```python
from build123d import *

# Parameters (mm, degrees)
ESQUISSE1_R = 1.25


with BuildPart() as part:
    # Balayage1: sweep along a path in Esquisse2
    with BuildLine(Plane(origin=(0, 0, 0), x_dir=(1, 0, 0), z_dir=(0, 1, 0))) as balayage1_path:
        Line((0, 0), (0, 5))
        ThreePointArc((0, 5), (-0.732233047, 6.767766953), (-2.5, 7.5))
        Line((-2.5, 7.5), (-25, 7.5))
        ThreePointArc((-25, 7.5), (-26.767766953, 6.767766953), (-27.5, 5))
        Line((-27.5, 5), (-27.5, -10))
        ThreePointArc((-27.5, -10), (-26.767766953, -11.767766953), (-25, -12.5))
        Line((-25, -12.5), (-2.5, -12.5))
        ThreePointArc((-2.5, -12.5), (-0.732233047, -11.767766953), (0, -10))
        Line((0, -10), (0, -5))
    # Esquisse1 → Balayage1 (sweep)
    with BuildSketch(Plane.XY):
        Circle(ESQUISSE1_R)
    sweep(path=balayage1_path.line)


solid = part.part
```
Build history of the part. All positions in model axes, mm. A direction names the side the tool comes from. Round coordinates to 2 decimals unless told otherwise and drop trailing zeros. Write each loop counter-clockwise with the first axis right and the second up, starting at its lowest first coordinate (ties: lowest second). Pieces come first, ordered by that corner, then holes. Notation, with made-up numbers: (43, 23) - (50, 23) arc R12 ccw to (50, 28) - close; hole circle Ø5 at (-22, 75). An arc over 180 degrees is marked (long way). Write each question's results on one line, items separated by ' | '. Start each with the question number.
Item 1: Wall check: L1, parallel to Z at x = -19, y = 0.05; L2, parallel to X at y = -0.1, z = -2.25; L3, parallel to Z at x = -24.5, y = -0.95. Give the ranges that are in metal, low to high. Write a range as [from, to].
Item 2: Saw through at B-B (z = 8). Write the cut outline in (x, y).
Item 3: Saw through at A-A (y = 0). Write the cut outline in (x, z), and give its area (3 significant figures).
Item 4: Saw through at C-C (x = -20). Write the cut outline in (y, z), and give its area (3 significant figures).
Item 5: Drop a flat-ended pin along its axis: P1, Ø1.2, axis at x = -0.5, y = 0.5, coming from the +Z side. Give the stop position or say it passes through.
Item 6: Saw through at D-D (z = 3). Write the cut outline in (x, y), and give its area (3 significant figures).
Item 7: Mould opens along X. For faces 1 (the face through (-13.91, -0.05, -6.25)), 2 (the face through (-13.59, -0.05, 11.25)), 3 (the face through (0, 0, 0)) say: pulls with the +X half, pulls with the -X half, needs draft (parallel to the pull), parting line crosses it, or undercut.
Item 8: Which spindle directions (+Z, -Z, +X, -X, +Y, -Y) get a long thin tool onto all of the face, cutting with end or side? Do faces 4 (the face through (0, 0, 5)), 5 (the face through (-0.27, 1.22, 7.46)). Say none if no direction does.
Results are:
1) L1: z = [-8.75, -6.25], [11.25, 13.75] | L2: x = [-28.75, -26.25], [-1.25, 1.25] | L3: z = [-8.31, -6.69], [11.69, 13.31]
2) outline: circle Ø2.5 at (-27.5, 0); circle Ø2.5 at (0, 0)
3) outline: (-28.75, -5) arc R3.75 ccw to (-25, -8.75) - (-2.5, -8.75) arc R3.75 ccw to (1.25, -5) - (1.25, 0) - (-1.25, 0) - (-1.25, -5) arc R1.25 cw to (-2.5, -6.25) - (-25, -6.25) arc R1.25 cw to (-26.25, -5) - (-26.25, 10) arc R1.25 cw to (-25, 11.25) - (-2.5, 11.25) arc R1.25 cw to (-1.25, 10) - (-1.25, 5) - (1.25, 5) - (1.25, 10) arc R3.75 ccw to (-2.5, 13.75) - (-25, 13.75) arc R3.75 ccw to (-28.75, 10) - close | area: 214 mm²
4) outline: circle Ø2.5 at (0, -7.5); circle Ø2.5 at (0, 12.5) | area: 9.82 mm²
5) P1: stops at z = 13.43
6) outline: circle Ø2.5 at (-27.5, 0) | area: 4.91 mm²
7) face 1: undercut | face 2: undercut | face 3: needs draft
8) face 4: +X, +Y, -Y | face 5: none
